Verification items for this drawing (mm, ordinates from the low corner). Round coordinates to 2 decimals unless told otherwise and drop trailing zeros. Loops run counter-clockwise (first coordinate to the right, second up) from the corner with the lowest first, then second, coordinate; pieces in that order, holes last. Notation, with made-up numbers: M 78.5,-33.75 L 109.5,-33.75 A29 cw 109.5,1.25 Z; hole C 36,50.25 d10. An arc over 180 degrees is marked long. Answer as CSV lines item,"result".
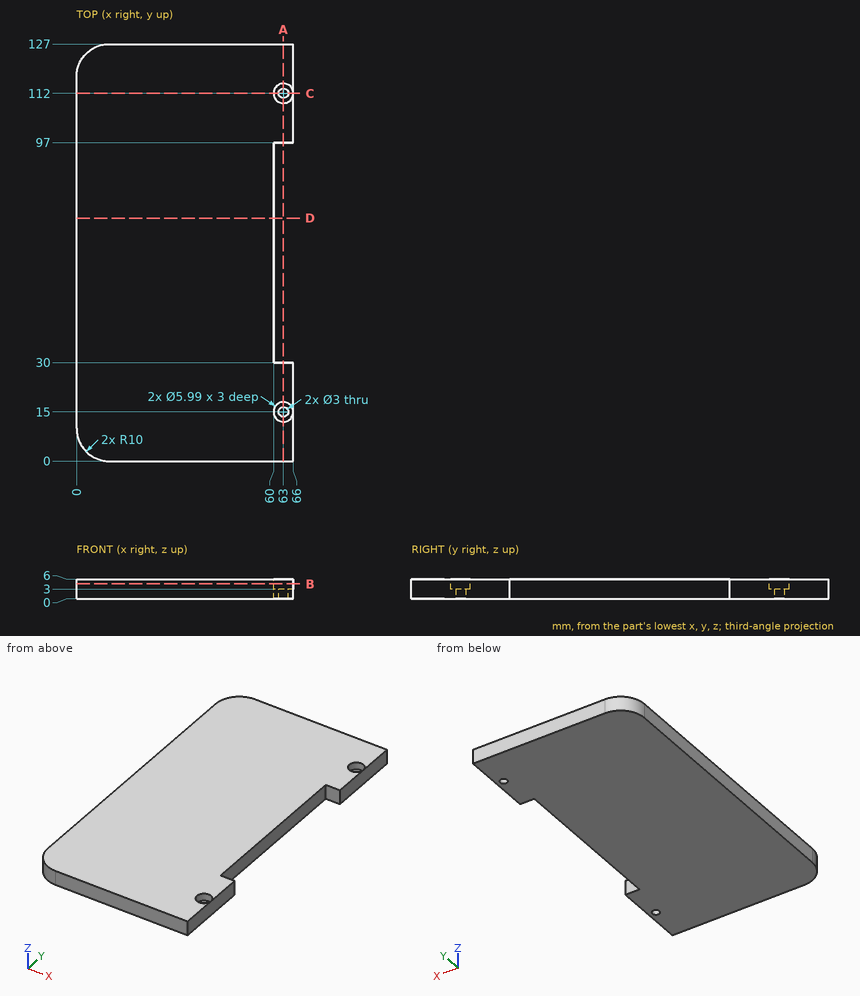
1) Go/stop test with flat-tipped pins: pin 1 (1.8 mm diameter, centred on y = 60.5, z = 3.5, fed in from +X); pin 2 (1.8 mm diameter, centred on x = 62.5, y = 14.5, fed in from +Z); pin 3 (1 mm diameter, centred on x = 28, y = 79.5, fed in from -Z); pin 4 (2.5 mm diameter, centred on x = 63, y = 15, fed in from +Z). Record where each tip stops, or that it passes through.
Here are the results:
pin 1,"stops at x = 60"
pin 2,"stops at z = 3"
pin 3,"stops at z = 0"
pin 4,"passes through"
2) Section check D-D (y = 74). Record the cut outline in (x, z).
Here are the results:
outline,"M 0,0 L 60,0 L 60,6 L 0,6 Z"
3) Section check A-A (x = 63). Record the cut outline in (y, z) (3 decimals).
Here are the results:
outline,"M 0,0 L 13.5,0 L 13.5,3 L 12.005,3 L 12.005,6 L 0,6 Z; M 16.5,0 L 30,0 L 30,6 L 17.995,6 L 17.995,3 L 16.5,3 Z; M 97,0 L 110.5,0 L 110.5,3 L 109.005,3 L 109.005,6 L 97,6 Z; M 113.5,0 L 127,0 L 127,6 L 114.995,6 L 114.995,3 L 113.5,3 Z"
4) Section check B-B (z = 4.6). Record the cut outline in (x, y) (3 decimals).
Here are the results:
outline,"M 0,10 A10 ccw 10,0 L 66,0 L 66,30 L 60,30 L 60,97 L 66,97 L 66,127 L 10,127 A10 ccw 0,117 Z; hole C 63,15 d5.99; hole C 63,112 d5.99"
5) Section check C-C (y = 112). Record the cut outline in (x, z) (3 decimals), plus the area to 3 significant figures.
Here are the results:
outline,"M 0,0 L 61.5,0 L 61.5,3 L 60.005,3 L 60.005,6 L 0,6 Z; M 64.5,0 L 66,0 L 66,6 L 65.995,6 L 65.995,3 L 64.5,3 Z"
area,"369 mm^2"
6) Material ranges on probe 1 along Y at (x, z) = (63, 4.2) (3 decimals); probe 2 along Y at (x, z) = (63, 1.9); probe 3 along X at (y, z) = (112, 1.6), recorded low to high.
Here are the results:
probe 1,"y = 0 to 12.005, 17.995 to 30, 97 to 109.005, 114.995 to 127"
probe 2,"y = 0 to 13.5, 16.5 to 30, 97 to 110.5, 113.5 to 127"
probe 3,"x = 0 to 61.5, 64.5 to 66"
